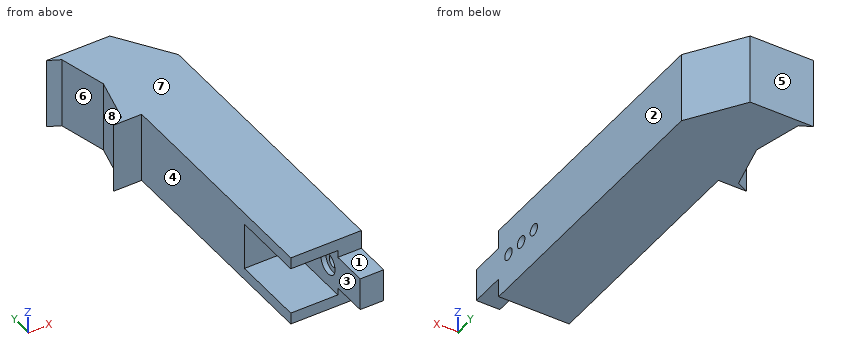
Autodesk Inventor part; units mm, degrees
ref_plane "YZ Plane" through (0, 0, 0) normal (1, 0, 0) x (0, 1, 0)
ref_plane "XZ Plane" through (0, 0, 0) normal (0, 1, 0) x (-1, 0, 0)
ref_plane "XY Plane" through (0, 0, 0) normal (0, 0, 1) x (1, 0, 0)
sketch "Sketch1" plane through (0, 0, 0) normal (0, 0, 1) x (1, 0, 0)
  line L0 (0, 0) -> (25, 0)
  line L1 (25, 0) -> (25, 40)
  line L2 (25, 40) -> (0, 40)
  line L3 (0, 40) -> (0, 0)
  dimension "d1" = 25
  dimension "d2" = 40
  dimension "d3" = 25
extrude "Extrusion1" add sketch "Sketch1" against normal blind 30
sketch "Sketch2" plane through (25, 0, 0) normal (1, 0, 0) x (0, 0, -1)
  line L0 (0, 0) -> (30, 0)
  circle A0 centre (15, 6.56) radius 2.46
extrude "Extrusion2" cut sketch "Sketch2" against normal blind 30
sketch "Sketch3" plane through (0, 0, 0) normal (-1, 0, 0) x (0, 0, 1)
  line L0 (0, 0) -> (-30, 0)
  line L1 (-25.05, 0) -> (-4.95, 0)
  line L2 (-4.95, 0) -> (-4.95, 33.12)
  line L3 (-4.95, 33.12) -> (-25.05, 33.12)
  line L4 (-25.05, 33.12) -> (-25.05, 0)
  dimension "d11" = 20.1
extrude "Extrusion3" cut sketch "Sketch3" against normal blind 20
sketch "Sketch4" plane through (0, 0, 0) normal (0, -1, 0) x (1, 0, 0)
  line L0 (20, -4.95) -> (20, -25.05)
  line L1 (20, -15) -> (25, -15)
  line L2 (25, 0) -> (25, -30)
  line L3 (20, -8.025) -> (25, -8.025)
  line L4 (25, -8.025) -> (25, -21.975)
  line L5 (25, -21.975) -> (20, -21.975)
  line L6 (20, -21.975) -> (20, -8.025)
  line L7 (20, -8.025) -> (25, -21.975) construction
  line L8 (25, -8.025) -> (20, -21.975) construction
  line L9 (25, -12.54) -> (25, -17.46)
  point P0 (0, 0)
  point P1 (22.5, -15)
  dimension "d14" = 13.95
extrude "Extrusion4" add sketch "Sketch4" along normal blind 15
sketch "Sketch5" plane through (20, 0, 0) normal (-1, 0, 0) x (0, 0, 1)
  circle A0 centre (-15, 6.56) radius 2.46
  circle A1 centre (-15, 6.56) radius 4.7025
  circle A2 centre (-15, 6.56) radius 2.46
  circle A3 centre (-15, 6.56) radius 2.46
  point P0 (0, 0)
  dimension "d17" = 9.405
extrude "Extrusion5" cut sketch "Sketch5" against normal blind 2.1
sketch "Sketch6" plane through (25, 0, 0) normal (1, 0, 0) x (0, 0, -1)
  circle A0 centre (15, 6.56) radius 4.7025
  line L0 (15, 6.56) -> (15, 23.56)
  circle A1 centre (15, 23.56) radius 2.46
  point P0 (0, 0)
  dimension "d20" = 17
  dimension "d21" = 4.92
extrude "Extrusion6" cut sketch "Sketch6" against normal blind 10 contours A1
sketch "Sketch7" plane through (20, 0, 0) normal (-1, 0, 0) x (0, 0, 1)
  circle A0 centre (-15, 23.56) radius 2.46
  circle A1 centre (-15, 23.56) radius 4.7025
  point P0 (0, 0)
  dimension "d24" = 9.405
extrude "Extrusion7" cut sketch "Sketch7" against normal blind 2.1
sketch "Sketch9" plane through (25, 0, 0) normal (1, 0, 0) x (0, 0, -1)
  circle A0 centre (15, 6.56) radius 2.46
  circle A1 centre (15, 6.56) radius 2.46
  circle A2 centre (15, 23.56) radius 2.46
  circle A3 centre (15, 23.56) radius 2.46
  line L0 (30, 40) -> (30, 0)
  line L1 (30, 0) -> (30, 40)
  line L2 (30, 40) -> (0, 40)
  line L3 (0, 40) -> (0, 0)
  line L4 (0, 0) -> (8.025, 0)
  line L5 (21.975, 0) -> (21.975, -15)
  line L6 (21.975, -15) -> (8.025, -15)
  line L7 (8.025, -15) -> (8.025, 0)
  line L8 (0, 0) -> (8.025, 0)
  line L9 (21.975, 0) -> (30, 0)
extrude "Extrusion8" add sketch "Sketch9" along normal blind 5
sketch "Sketch10" plane through (0, 40, 0) normal (0, 1, 0) x (1, 0, 0)
  line L0 (0, 30) -> (30, 30)
  line L1 (30, 0) -> (0, 0)
  line L2 (0, 30) -> (30, 30)
  line L3 (30, 30) -> (30, 0)
  line L4 (30, 0) -> (0, 0)
  line L5 (0, 0) -> (0, 30)
extrude "Extrusion9" add sketch "Sketch10" along normal blind 30
sketch "Sketch12" plane through (30, 0, 0) normal (1, 0, 0) x (0, 0, -1)
  circle A0 centre (15, 6.56) radius 2.46
  line L0 (15, 6.56) -> (15, 15.06)
  circle A1 centre (15, 15.06) radius 2.525
  point P0 (0, 0)
  dimension "d31" = 8.5
  dimension "d33" = 5.05
extrude "Extrusion10" cut sketch "Sketch12" against normal blind 30 contours A1
sketch "Sketch14" plane through (0, 0, 0) normal (0, 0, 1) x (1, 0, 0)
  line L0 (30, 70) -> (0, 70)
  line L1 (0, 70) -> (0, 100)
  line L2 (30, 0) -> (30, 70)
  line L3 (30, 122.5) -> (30, 70)
  line L4 (30, 105) -> (30, 100)
  line L5 (-12, 145) -> (15, 145)
  line L6 (-7, 142.5) -> (-12, 145)
  line L7 (-7, 102.5) -> (-12, 100)
  line L8 (-7, 102.5) -> (-2, 122.5)
  line L9 (-2, 122.5) -> (-7, 142.5)
  line L10 (30, 122.5) -> (15, 145)
  line L11 (0, 100) -> (-12, 100)
  point P0 (0, 0)
  dimension "d86" = 12
extrude "Extrusion12" add sketch "Sketch14" against normal blind 30
sketch "Sketch15" plane through (0, 0, -25.05) normal (-1, 0, 0) x (0, 0, 1)
  line L0 (0, 33.12) -> (20.1, 33.12)
  line L1 (20.1, 33.12) -> (20.1, 0)
  line L2 (0, 33.12) -> (20.1, 33.12)
  line L3 (20.1, 33.12) -> (20.1, 31.1)
  line L4 (20.1, 31.1) -> (0, 31.1)
  line L5 (0, 31.1) -> (0, 33.12)
  point P0 (25.05, 0)
  dimension "d57" = 2.02
extrude "Extrusion13" add sketch "Sketch15" against normal blind 20
properties part number "rec_a_40mm_x_30mm"
Check sheet for the modelled part. Datum: model origin and axes. Units: mm. Face numbers are marked on the shaded views. A direction names the side the tool comes from. Round coordinates to 2 decimals unless told otherwise and drop trailing zeros. Order: outer loops, then holes, each group sorted by start corner. A loop starts at its lowest first (then second) coordinate and runs counter-clockwise, first axis right, second up. Notation, with made-up numbers: M 67,-31 L 77,-31 A17 ccw 77,-5 Z; hole C 36,22.25 d2. An arc over 180 degrees is marked long. Answer in a Markdown table with one row per item.
(1) Draft check along Y on the marked faces 5, 6, 7 and 8. Enter one of: +Y half, -Y half, draft (parallel to the pull), parting line (faces both ways), or undercut.
Findings:
| item | result |
|---|---|
| face 5 | +Y half |
| face 6 | undercut |
| face 7 | draft |
| face 8 | undercut |
(2) Material ranges on line 1 along Y through (x, z) = (27, -15) (3 decimals); line 2 along Y through (x, z) = (21.35, -15) (1 decimal); line 3 along Z through (x, y) = (26.5, 15.06) (3 decimals), recorded low to high. Write a range as from..to.
Findings:
| item | result |
|---|---|
| line 1 | y = -15..4.1, 9.02..12.535, 17.585..21.1, 26.02..127 |
| line 2 | y = -15..1.9, 11.3..12.5, 17.6..18.9, 28.3..135.5 |
| line 3 | z = -30..-17.525, -12.475..0 |
(3) Section check B-B on x = 27. Record the boundary of the cut face in (y, z) (3 decimals).
Findings:
| item | result |
|---|---|
| outline | M -15,-21.975 L 0,-21.975 L 0,-30 L 127,-30 L 127,0 L 0,0 L 0,-8.025 L -15,-8.025 Z; hole C 6.56,-15 d4.92; hole C 15.06,-15 d5.05; hole C 23.56,-15 d4.92 |
(4) Gauge pin test, flat ends, axial feed: pin 1 (12 mm diameter, centred on y = 63, z = -6, fed in from -X); pin 2 (3 mm diameter, centred on y = 6.5, z = -15.5, fed in from -X); pin 3 (6 mm diameter, centred on x = -5, z = -8, fed in from -Y); pin 4 (5 mm diameter, centred on x = 25.5, y = -10.5, fed in from +Z) (3 decimals). Record the tip position at first contact, or that the pin passes through.
Findings:
| item | result |
|---|---|
| pin 1 | stops at x = 0 |
| pin 2 | passes through |
| pin 3 | stops at y = 100 |
| pin 4 | stops at z = -8.025 |
(5) Section check D-D on x = 6.5. Record the boundary of the cut face in (y, z).
Findings:
| item | result |
|---|---|
| outline | M 0,-30 L 145,-30 L 145,0 L 0,0 L 0,-4.95 L 31.1,-4.95 L 31.1,-25.05 L 0,-25.05 Z |
(6) Section check A-A on z = -15. Give the number of separate pieces and of enclosed holes in the cut face, plus the area to 3 significant figures.
Findings:
| item | result |
|---|---|
| separate pieces | 4 |
| enclosed holes | 0 |
| area | 3,770 mm^2 |
(7) Section check C-C on y = 15.06. Record the boundary of the cut face in (x, z) (3 decimals).
Findings:
| item | result |
|---|---|
| outline | M 0,-30 L 30,-30 L 30,-17.525 L 20,-17.525 L 20,-25.05 L 0,-25.05 Z; M 0,-4.95 L 20,-4.95 L 20,-12.475 L 30,-12.475 L 30,0 L 0,0 Z |
(8) Set-up check for the marked faces 1, 2, 3 and 4: record each of +Z, -Z, +X, -X, +Y, -Y from which the full face is reachable in a straight line by a thin tool's end or side.
Findings:
| item | result |
|---|---|
| face 1 | +Z, +X, -X, -Y |
| face 2 | +Z, -Z, +X, +Y, -Y |
| face 3 | -X, -Y |
| face 4 | +Z, -Z, -X, -Y |
